Geometry: final body of the model. Coordinates: model frame, mm. Round coordinates to 2 decimals unless told otherwise and drop trailing zeros. Loops run counter-clockwise (first coordinate to the right, second up) from the corner with the lowest first, then second, coordinate; pieces in that order, holes last. Notation, with made-up numbers: (13, -37.75) -> (33, -37.75) arc R19 ccw to (33, -8.75) -> close; hole circle Ø7 at (89, 50.5). An arc over 180 degrees is marked (long way). Answer in a Markdown table with one row per item.
```python
from build123d import *

# Parameters (mm, degrees)
SKETCH1_R                         = 23
LENGTH_DEPTH                      = 505
FEMUR_HOLE_REACH                  = 508.046
FEMUR_HOLE_END_RADIUS             = 23
SKETCH2_R                         = 8.430886207
SKETCH2_R_2                       = 10.877092796
FEMUR_HOLE_DIRECTION_2_REACH      = 508.046
FEMUR_HOLE_DIRECTION_2_END_RADIUS = 23


with BuildPart() as part:
    # Sketch1 → Length (new body)
    with BuildSketch(Plane(origin=(0, 0, 0), x_dir=(0, 0, -1), z_dir=(1, 0, 0))):
        Circle(SKETCH1_R)
    extrude(amount=LENGTH_DEPTH)

    # Femur hole: up to this cylinder (the profile starts inside it)
    femur_hole_end = Plane(origin=(254.436174, 0, 0), z_dir=(-1, 0, 0)) * Cylinder(FEMUR_HOLE_END_RADIUS, 1571.964348, mode=Mode.PRIVATE)
    # Sketch2 → Femur hole (cut, up to the surface)
    with BuildSketch(Plane.XY, mode=Mode.PRIVATE) as femur_hole_sk1:
        Circle(SKETCH2_R)
    femur_hole_tool1 = extrude(femur_hole_sk1.sketch, amount=-FEMUR_HOLE_REACH, mode=Mode.PRIVATE) & femur_hole_end
    add(femur_hole_tool1.solids().sort_by_distance((0, 0, 0))[0], mode=Mode.SUBTRACT)
    # Sketch2 → Femur hole (cut, up to the surface)
    with BuildSketch(Plane.XY, mode=Mode.PRIVATE) as femur_hole_sk2:
        with Locations((508.872347898, 0)):
            Circle(SKETCH2_R_2)
    femur_hole_tool2 = extrude(femur_hole_sk2.sketch, amount=-FEMUR_HOLE_REACH, mode=Mode.PRIVATE) & femur_hole_end
    add(femur_hole_tool2.solids().sort_by_distance((508.872348, 0, 0))[0], mode=Mode.SUBTRACT)

    # Femur hole direction 2: up to this cylinder (the profile starts inside it)
    femur_hole_direction_2_end = Plane(origin=(254.436174, 0, 0), z_dir=(-1, 0, 0)) * Cylinder(FEMUR_HOLE_DIRECTION_2_END_RADIUS, 1571.964348, mode=Mode.PRIVATE)
    # Sketch2 → Femur hole direction 2 (cut, up to the surface)
    with BuildSketch(Plane.XY, mode=Mode.PRIVATE) as femur_hole_direction_2_sk1:
        Circle(SKETCH2_R)
    femur_hole_direction_2_tool1 = extrude(femur_hole_direction_2_sk1.sketch, amount=FEMUR_HOLE_DIRECTION_2_REACH, mode=Mode.PRIVATE) & femur_hole_direction_2_end
    add(femur_hole_direction_2_tool1.solids().sort_by_distance((0, 0, 0))[0], mode=Mode.SUBTRACT)
    # Sketch2 → Femur hole direction 2 (cut, up to the surface)
    with BuildSketch(Plane.XY, mode=Mode.PRIVATE) as femur_hole_direction_2_sk2:
        with Locations((508.872347898, 0)):
            Circle(SKETCH2_R_2)
    femur_hole_direction_2_tool2 = extrude(femur_hole_direction_2_sk2.sketch, amount=FEMUR_HOLE_DIRECTION_2_REACH, mode=Mode.PRIVATE) & femur_hole_direction_2_end
    add(femur_hole_direction_2_tool2.solids().sort_by_distance((508.872348, 0, 0))[0], mode=Mode.SUBTRACT)


solid = part.part
```
Item 1: Section query C-C, the plane x = 108.5. Output: boundary loops of the cut face in (y, z), and give its area (3 significant figures).
Ans:
| item | result |
|---|---|
| outline | circle Ø46 at (0, 0) |
| area | 1,660 mm2 |
Item 2: Section query D-D, the plane z = 13. Output: boundary loops of the cut face in (x, y), and give its area (3 significant figures).
Ans:
| item | result |
|---|---|
| outline | (0, -18.97) -> (505, -18.97) -> (505, -10.16) arc R10.88 cw to (505, 10.16) -> (505, 18.97) -> (0, 18.97) -> (0, 8.43) arc R8.43 cw to (0, -8.43) -> close |
| area | 18,900 mm2 |
Item 3: Section query B-B, the plane y = 0. Output: boundary loops of the cut face in (x, z), and give its area (3 significant figures).
Ans:
| item | result |
|---|---|
| outline | (8.43, -23) -> (498, -23) -> (498, 23) -> (8.43, 23) -> close |
| area | 22,500 mm2 |
Item 4: First-contact query: P1, Ø3, axis at y = 2.5, z = -6, coming from the -X side; P2, Ø6, axis at x = 202.5, z = 4.5, coming from the +Y side; P3, Ø4, axis at y = -1, z = -2.5, coming from the -X side. Flat tips, straight axial feed; report the tip coordinate or a pass-through.
Ans:
| item | result |
|---|---|
| P1 | x = 7.42 |
| P2 | y = 22.95 |
| P3 | x = 7.88 |
Item 5: Mould query, pull axis Y, two halves, no side actions, for faces 1 (the cylindrical face through (8.43, -0.19, 0.32)), 2 (the flat face through (0, -14, 0)), 3 (the cylindrical face through (248.965, 22.804, 2.994)). Classes: released by +Y, released by -Y, zero draft, split by the parting line, or undercut.
Ans:
| item | result |
|---|---|
| face 1 | undercut |
| face 2 | zero draft |
| face 3 | split by the parting line |
Item 6: Section query A-A, the plane z = -7. Output: boundary loops of the cut face in (x, y).
Ans:
| item | result |
|---|---|
| outline | (0, -21.91) -> (505, -21.91) -> (505, -10.16) arc R10.88 cw to (505, 10.16) -> (505, 21.91) -> (0, 21.91) -> (0, 8.43) arc R8.43 cw to (0, -8.43) -> close |
Item 7: Ray query, L1, parallel to X at y = 0.5, z = 5; L2, parallel to Y at x = 445, z = 1; L3, parallel to Y at x = 114.5, z = -2. Return the intervals inside material, ascending.
Ans:
| item | result |
|---|---|
| L1 | 8.42 to 498.01 |
| L2 | -22.98 to 22.98 |
| L3 | -22.91 to 22.91 |
